```python
from build123d import *

# Parameters (mm, degrees)
SKETCH1_W           = 2100
SKETCH1_H           = 1178.5
SKETCH1_W_2         = 1980
SKETCH1_H_2         = 1000
BOSS_EXTRUDE1_DEPTH = 30
SKETCH2_R           = 6.35
CUT_EXTRUDE1_DEPTH  = 1205.415029174


with BuildPart() as part:
    # Sketch1 → Boss-Extrude1 (new body)
    with BuildSketch(Plane(origin=(0, 0, 0), x_dir=(1, 0, 0), z_dir=(0, 1, 0))):
        Rectangle(SKETCH1_W, SKETCH1_H)
        with Locations((0, 5)):
            Rectangle(SKETCH1_W_2, SKETCH1_H_2, mode=Mode.SUBTRACT)
    extrude(amount=-BOSS_EXTRUDE1_DEPTH)

    # Sketch2 → Cut-Extrude1 (cut, through all)
    with BuildSketch(Plane(origin=(0, 0, 0), x_dir=(1, 0, 0), z_dir=(0, 1, 0))):
        with Locations(Location((-1020, 559.25, 0), (0, 0, 270))):
            Circle(SKETCH2_R)
        with Locations(Location((-1020, -559.25, 0), (0, 0, 270))):
            Circle(SKETCH2_R)
        with Locations(Location((1020, 559.25, 0), (0, 0, 270))):
            Circle(SKETCH2_R)
        with Locations(Location((1020, -559.25, 0), (0, 0, 270))):
            Circle(SKETCH2_R)
    extrude(amount=-CUT_EXTRUDE1_DEPTH, mode=Mode.SUBTRACT)


solid = part.part
```
Geometry check sheet. Reference: the model listing, model coordinates, mm. Give positions to 0.01 mm unless a question says otherwise; leave off trailing zeros. Order: outer loops, then holes, each group sorted by start corner. A loop starts at its lowest first (then second) coordinate and runs counter-clockwise, first axis right, second up.
1. Section check A-A, the plane x = -384. Enter the section's corners in (y, z), and give its area (4 significant figures).
2. Thickness scan on L1, parallel to Z at x = 1020, y = -11.5; L2, parallel to X at y = -15, z = -559.25; L3, parallel to X at y = -25.75, z = -386. Record the ranges inside material, lowest first.
3. Section check B-B, the plane y = -19.25. Enter the section's corners in (x, z).
4. Section check C-C, the plane z = 381. Enter the section's corners in (x, y).
5. Gauge pin test, flat end, axial feed: pin 1 Ø11.5 at (x, z) = (-1020, 559.25) entering from +Y. Record the tip position at first contact, or that the pin passes through.
Values follow:
1. outline: (-30, -589.25) - (0, -589.25) - (0, -505) - (-30, -505) - close; (-30, 495) - (0, 495) - (0, 589.25) - (-30, 589.25) - close
1. area: 5,355 mm2
2. L1: z = -589.25 to -565.6, -552.9 to 552.9, 565.6 to 589.25
2. L2: x = -1050 to -1026.35, -1013.65 to 1013.65, 1026.35 to 1050
2. L3: x = -1050 to -990, 990 to 1050
3. outline: (-1050, -589.25) - (1050, -589.25) - (1050, 589.25) - (-1050, 589.25) - close; hole circle Ø12.7 at (-1020, -559.25); hole circle Ø12.7 at (-1020, 559.25); hole (-990, -505) - (990, -505) - (990, 495) - (-990, 495) - close; hole circle Ø12.7 at (1020, -559.25); hole circle Ø12.7 at (1020, 559.25)
4. outline: (-1050, -30) - (-990, -30) - (-990, 0) - (-1050, 0) - close; (990, -30) - (1050, -30) - (1050, 0) - (990, 0) - close
5. pin 1: passes through
